```python
from build123d import *

# Parameters (mm, degrees)
SKETCH1_R               = 15
SKETCH1_R_2             = 7.5
BOSS_EXTRUDE1_DEPTH     = 3
SKETCH2_R               = 11
SKETCH2_R_2             = 7.5
BOSS_EXTRUDE2_DEPTH     = 6
CUT_EXTRUDE1_DEPTH      = 24.043437244
CUT_EXTRUDE1_DEPTH_BACK = 24.043437244
SKETCH3_R               = 1.75


with BuildPart() as part:
    # Sketch1 → Boss-Extrude1 (new body)
    with BuildSketch(Plane(origin=(0, 0, 0), x_dir=(1, 0, 0), z_dir=(0, 1, 0))):
        with Locations(Location((0, 0, 0), (0, 0, 270))):
            Circle(SKETCH1_R)
        with Locations(Location((0, 0, 0), (0, 0, 270))):
            Circle(SKETCH1_R_2, mode=Mode.SUBTRACT)
    extrude(amount=BOSS_EXTRUDE1_DEPTH)

    # Sketch2 → Boss-Extrude2 (add)
    with BuildSketch(Plane(origin=(0, 3, 0), x_dir=(1, 0, 0), z_dir=(0, 1, 0))):
        with Locations(Location((0, 0, 0), (0, 0, 270))):
            Circle(SKETCH2_R)
        with Locations(Location((0, 0, 0), (0, 0, 270))):
            Circle(SKETCH2_R_2, mode=Mode.SUBTRACT)
    extrude(amount=BOSS_EXTRUDE2_DEPTH)

    # Sketch3 → Cut-Extrude1 (cut, two sides: drawn at the far end of the back side and taken through both)
    with BuildSketch(Plane.XY.offset(-CUT_EXTRUDE1_DEPTH_BACK)):
        with Locations((0, 6)):
            Circle(SKETCH3_R)
    extrude(amount=CUT_EXTRUDE1_DEPTH + CUT_EXTRUDE1_DEPTH_BACK, mode=Mode.SUBTRACT)


solid = part.part
```
CAD build for the part. Positions are in the model's coordinates, mm. A direction names the side the tool comes from. Round coordinates to 2 decimals unless told otherwise and drop trailing zeros. Order: outer loops, then holes, each group sorted by start corner. A loop starts at its lowest first (then second) coordinate and runs counter-clockwise, first axis right, second up. Notation, with made-up numbers: (-36.75, 81.25) -> (-10.75, 81.25) arc R10 cw to (-10.75, 89.25) -> close; hole circle Ø9 at (74.25, -31.5). An arc over 180 degrees is marked (long way). Write item = value, one per line.
(1) 3-axis set-ups, long thin cutter, end or side, ignore diameter. For faces 1 (the cylindrical face through (-2.87, 4.44, 6.93)), 2 (the cylindrical face through (-4.213, 5.958, 10.161)): which of +Z, -Z, +X, -X, +Y, -Y reach the whole face in a straight line?
Answers follow:
face_1 = +Y, -Y
face_2 = +Y
(2) Cut at D-D (z = 8.25). Write the cut outline in (x, y), plus the area to 3 significant figures.
Answers follow:
outline = (-12.53, 0) -> (12.53, 0) -> (12.53, 3) -> (7.28, 3) -> (7.28, 9) -> (-7.28, 9) -> (-7.28, 3) -> (-12.53, 3) -> close; hole circle Ø3.5 at (0, 6)
area = 153 mm²
(3) Drill centre lines: L1, parallel to X at y = 6, z = -8.05; L2, parallel to X at y = 4.5, z = 0; L3, parallel to Y at x = 0, z = 8.75. Where is each one in solid material? Low to high.
Answers follow:
L1 = -7.5 to -1.75, 1.75 to 7.5
L2 = -11 to -7.5, 7.5 to 11
L3 = 0 to 4.25, 7.75 to 9
(4) Pull direction Y, two halves, no side cores. Call faces 3 (the cylindrical face through (-0.38, 4.29, -9.17)), 4 (the flat face through (10, 3, -5)), 5 (the flat face through (7, 0, -4)): +Y half, -Y half, draft (parallel to the pull), parting line (faces both ways), or undercut.
Answers follow:
face_3 = undercut
face_4 = +Y half
face_5 = -Y half
(5) Flat gauge pins, fed straight in: P1, Ø3, axis at x = 11, z = -9, coming from the -Y side; P2, Ø4, axis at x = 8, z = 10.5, coming from the +Y side; P3, Ø4, axis at y = 3.5, z = -11.5, coming from the +X side; P4, Ø1.5, axis at y = 6, z = 0.5, coming from the +X side. Where does each tip first touch, or does it go through?
Answers follow:
P1 = 0
P2 = 3
P3 = 11.56
P4 = 11
(6) Cut at C-C (y = 6). Write the cut outline in (x, z), plus the area to 3 significant figures.
Answers follow:
outline = (-1.75, -10.86) -> (-1.75, -7.29) arc R7.5 cw to (-1.75, 7.29) -> (-1.75, 10.86) arc R11 ccw to start; (1.75, -10.86) arc R11 ccw to (1.75, 10.86) -> (1.75, 7.29) arc R7.5 cw to (1.75, -7.29) -> close
area = 179 mm²
(7) Cut at A-A (x = 0). Write the cut outline in (y, z).
Answers follow:
outline = (0, -15) -> (3, -15) -> (3, -11) -> (4.25, -11) -> (4.25, -7.5) -> (0, -7.5) -> close; (0, 7.5) -> (4.25, 7.5) -> (4.25, 11) -> (3, 11) -> (3, 15) -> (0, 15) -> close; (7.75, -11) -> (9, -11) -> (9, -7.5) -> (7.75, -7.5) -> close; (7.75, 7.5) -> (9, 7.5) -> (9, 11) -> (7.75, 11) -> close
(8) Cut at B-B (z = 0). Write the cut outline in (x, y), plus the area to 3 significant figures.
Answers follow:
outline = (-15, 0) -> (-7.5, 0) -> (-7.5, 9) -> (-11, 9) -> (-11, 3) -> (-15, 3) -> close; (7.5, 0) -> (15, 0) -> (15, 3) -> (11, 3) -> (11, 9) -> (7.5, 9) -> close
area = 87.0 mm²
